Verification items for the finished model (mm, model axes). A direction names the side the tool comes from. Coordinates: 2 decimals unless noted, no trailing zeros. Write each loop counter-clockwise with the first axis right and the second up, starting at its lowest first coordinate (ties: lowest second). Pieces come first, ordered by that corner, then holes.
```python
from build123d import *

# Parameters (mm, degrees)
F0_W     = 355.6
F0_H     = 152.4
F1_DEPTH = 3.175
F2_W     = 44.45
F2_H     = 44.45
F3_DEPTH = 203.2
F5_D     = 15.875


with BuildPart() as f1:
    # F0 (on Top) → F1 (new body)
    with BuildSketch(Plane.XY):
        Rectangle(F0_W, F0_H)
    extrude(amount=F1_DEPTH)

    # F2 (on Front) → F3 (join)
    with BuildSketch(Plane.XZ):
        with BuildLine():
            Line((22.225, 0), (-22.225, 0))
            ThreePointArc((-22.225, 0), (-24.470064, -0.929936), (-25.4, -3.175))
            Line((-25.4, -3.175), (-25.4, -47.625))
            ThreePointArc((-25.4, -47.625), (-24.470064, -49.870064), (-22.225, -50.8))
            Line((-22.225, -50.8), (22.225, -50.8))
            ThreePointArc((22.225, -50.8), (24.470064, -49.870064), (25.4, -47.625))
            Line((25.4, -47.625), (25.4, -3.175))
            ThreePointArc((25.4, -3.175), (24.470064, -0.929936), (22.225, 0))
        make_face()
        with Locations((0, -25.4)):
            Rectangle(F2_W, F2_H, mode=Mode.SUBTRACT)
    extrude(amount=-F3_DEPTH)

    # F5 (through all)
    with Locations(Plane(origin=(-25.4, 0, 0), x_dir=(0, -1, 0), z_dir=(-1, 0, 0))):
        with Locations((-152.4, -25.4)):
            Hole(F5_D / 2)


solid = f1.part
```
1. Gauge pin test, flat ends, axial feed: P1, Ø4, axis at x = -106, y = 61, coming from the -Z side; P2, Ø2.5, axis at x = -31, z = 2, coming from the +Y side; P3, Ø3, axis at y = 18.5, z = -16.5, coming from the -X side; P4, Ø14.5, axis at y = 152.4, z = -25.4, coming from the -X side. Record the tip position at first contact, or that the pin passes through.
2. Sectioned sample at D-D, the plane y = 115.5. Record the boundary of the cut face in (x, z) (3 decimals), and give its area (3 significant figures).
3. Material ranges on L1, parallel to X at y = 192.5, z = -37 (3 decimals); L2, parallel to Z at x = 74, y = 8 (3 decimals); L3, parallel to Z at x = -23.1, y = 152.4, recorded low to high.
4. Tool access check on faces 1 (the flat face through (0, 139, 0)), 2 (the flat face through (-22.225, 100, -26)), 3 (the flat face through (-25.4, 100, -25)), 4 (the flat face through (25.4, 100, -26)), 5 (the flat face through (-2, 1, 3.175)). Record the directions out of +Z, -Z, +X, -X, +Y, -Y that give a thin tool (end or side, any length) a straight path to the whole face; none if there is none.
5. Sectioned sample at C-C, the plane y = 12.5. Record the boundary of the cut face in (x, z) (3 decimals).
6. Sectioned sample at A-A, the plane z = -11. Record the boundary of the cut face in (x, y) (3 decimals).
7. Draft check along Y on faces 6 (the flat face through (0, 100, -47.625)), 7 (the flat face through (2, 0, -48)), 8 (the cylindrical face through (-23.79, 159.971, -23.016)), 9 (the cylindrical face through (23.835, 159.971, -23.016)). Enter one of: pulls with the +Y half, pulls with the -Y half, needs draft (parallel to the pull), parting line crosses it, or undercut.
Outcome:
1. P1: stops at z = 0
1. P2: stops at y = 76.2
1. P3: stops at x = -25.4
1. P4: passes through
2. outline: (-25.4, -47.625) arc R3.175 ccw to (-22.225, -50.8) - (22.225, -50.8) arc R3.175 ccw to (25.4, -47.625) - (25.4, -3.175) arc R3.175 ccw to (22.225, 0) - (-22.225, 0) arc R3.175 ccw to (-25.4, -3.175) - close; hole (-22.225, -47.625) - (22.225, -47.625) - (22.225, -3.175) - (-22.225, -3.175) - close
2. area: 596 mm2
3. L1: x = -25.4 to -22.225, 22.225 to 25.4
3. L2: z = 0 to 3.175
3. L3: z = -50.68 to -33.34, -17.46 to -0.12
4. face 1: +Z, +X, -X, +Y
4. face 2: +Y, -Y
4. face 3: -Z, -X, +Y, -Y
4. face 4: -Z, +X, +Y, -Y
4. face 5: +Z, +X, -X, +Y, -Y
5. outline: (-177.8, 0) - (-22.225, 0) arc R3.175 ccw to (-25.4, -3.175) - (-25.4, -47.625) arc R3.175 ccw to (-22.225, -50.8) - (22.225, -50.8) arc R3.175 ccw to (25.4, -47.625) - (25.4, -3.175) arc R3.175 ccw to (22.225, 0) - (177.8, 0) - (177.8, 3.175) - (-177.8, 3.175) - close; hole (-22.225, -47.625) - (22.225, -47.625) - (22.225, -3.175) - (-22.225, -3.175) - close
6. outline: (-25.4, 0) - (-22.225, 0) - (-22.225, 203.2) - (-25.4, 203.2) - close; (22.225, 0) - (25.4, 0) - (25.4, 203.2) - (22.225, 203.2) - close
7. face 6: needs draft
7. face 7: pulls with the -Y half
7. face 8: undercut
7. face 9: undercut
